Part print with two shaded views. Sizes in mm from the minimum x, y, z corner. Round coordinates to 2 decimals unless told otherwise and drop trailing zeros. Write each loop counter-clockwise with the first axis right and the second up, starting at its lowest first coordinate (ties: lowest second). Pieces come first, ordered by that corner, then holes. Notation, with made-up numbers: (54, -29.5) -> (104, -29.5) arc R26 cw to (104, 3.5) -> close; hole circle Ø5 at (-0.75, 61.25). An arc over 180 degrees is marked (long way). Return JSON: item names as keys, results as strings. Group by question number.
(1) Drop a flat-ended pin along its axis: pin 1 Ø11 at (x, z) = (166, 67) entering from +Y. Give the stop position or say it passes through.
(2) Saw through at C-C (y = 1.8). List the corners of the cut face in (x, z), plus the area to 3 significant figures.
(3) Saw through at A-A (z = 67). List the corners of the cut face in (x, y), plus the area to 3 significant figures.
(4) Drill centre lines: L1, parallel to Z at x = 166, y = 2.2; L2, parallel to X at y = 1.35, z = 22; L3, parallel to Z at x = 14, y = 1.7. Where is each one in solid material? Low to high. Write a range as from..to.
(5) Saw through at B-B (x = 166). List the corners of the cut face in (y, z), plus the area to 3 significant figures.
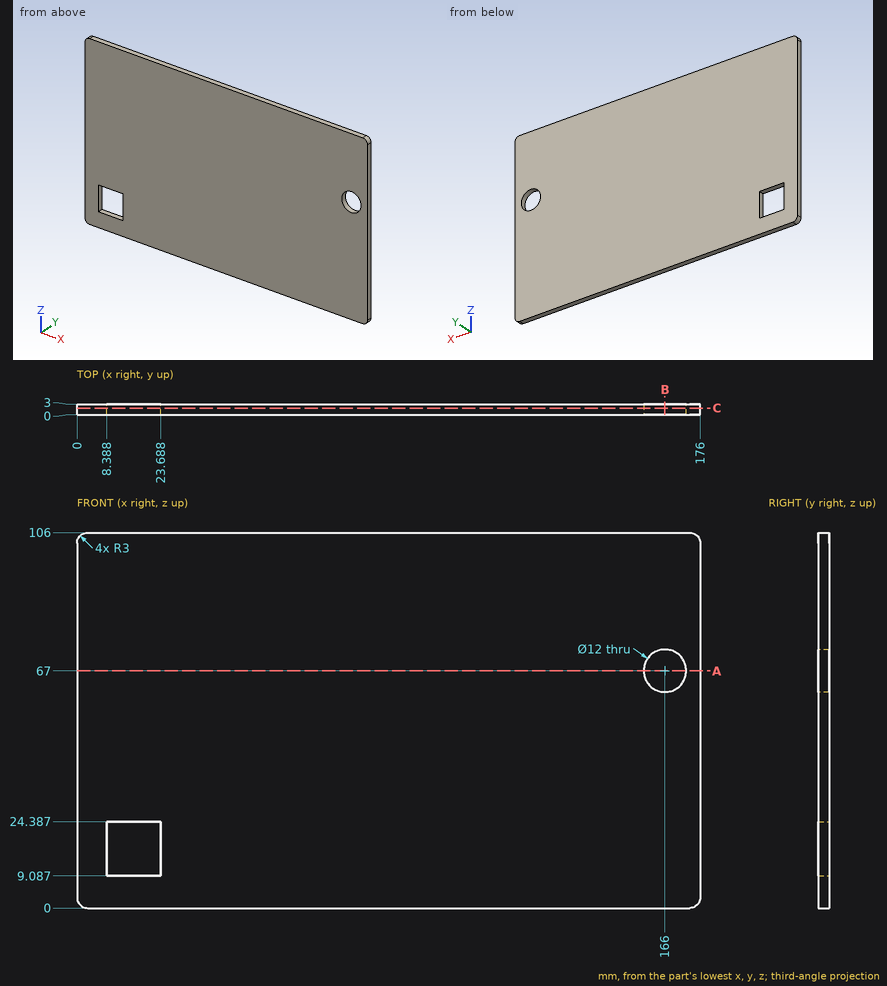
Computed values:
{
 "1": {"pin 1": "through"},
 "2": {"outline": "(0, 3) arc R3 ccw to (3, 0) -> (173, 0) arc R3 ccw to (176, 3) -> (176, 103) arc R3 ccw to (173, 106) -> (3, 106) arc R3 ccw to (0, 103) -> close; hole (8.39, 9.09) -> (23.69, 9.09) -> (23.69, 24.39) -> (8.39, 24.39) -> close; hole circle Ø12 at (166, 67)", "area": "18,300 mm2"},
 "3": {"outline": "(0, 0) -> (160, 0) -> (160, 3) -> (0, 3) -> close; (172, 0) -> (176, 0) -> (176, 3) -> (172, 3) -> close", "area": "492 mm2"},
 "4": {"L1": "0..61, 73..106", "L2": "0..8.39, 23.69..176", "L3": "0..9.09, 24.39..106"},
 "5": {"outline": "(0, 0) -> (3, 0) -> (3, 61) -> (0, 61) -> close; (0, 73) -> (3, 73) -> (3, 106) -> (0, 106) -> close", "area": "282 mm2"}
}
